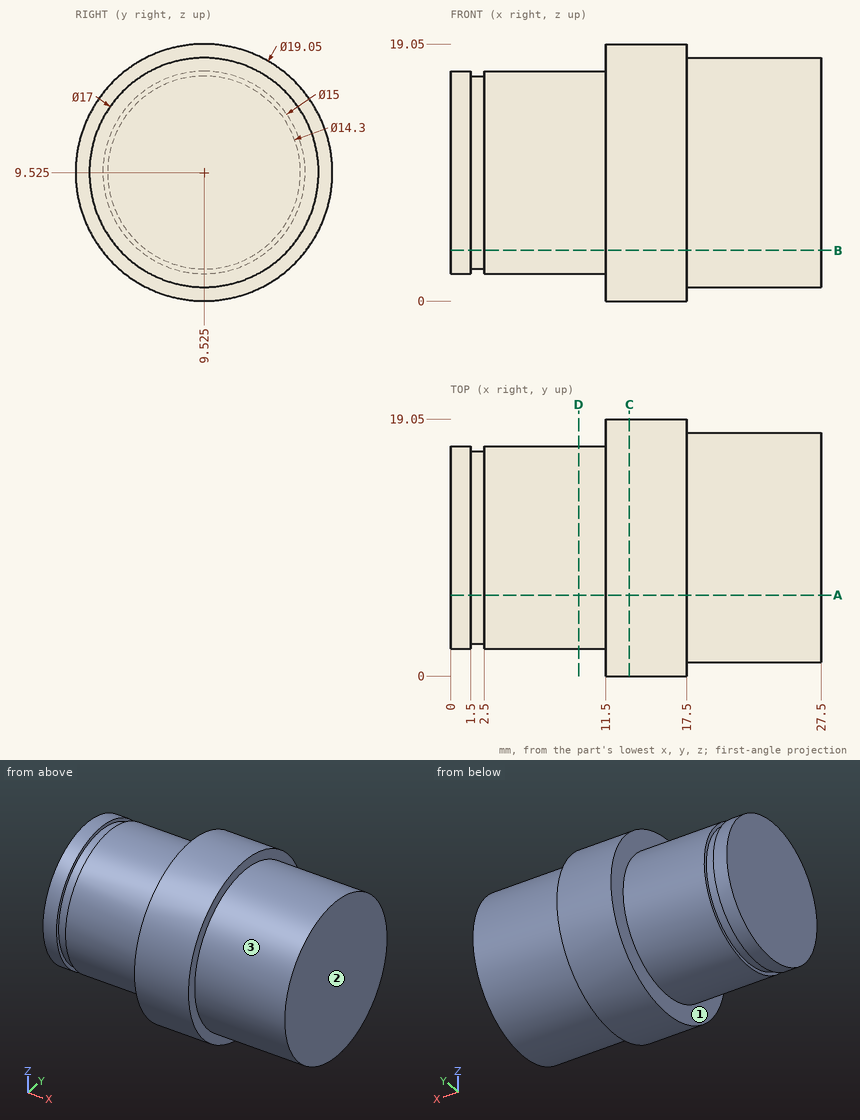
Geometry: see drawing. Coordinates: mm, zero at the bounding-box minimum. A direction names the side the tool comes from. Coordinates: 2 decimals unless noted, no trailing zeros. Loops run counter-clockwise (first coordinate to the right, second up) from the corner with the lowest first, then second, coordinate; pieces in that order, holes last. Notation, with made-up numbers: (-16.5, -16.5) - (17.5, -16.5) arc R22 ccw to (17.5, 19.5) - close; hole circle Ø3 at (3.25, 21). An arc over 180 degrees is marked (long way). Put each result on its own line as item: value. Start each with the question number.
Q1. Cut plane A-A, the plane y = 6. Return loops of the section in (x, z) (3 decimals).
Q2. Set-up query: the marked faces 1, 2 and 3. Return all of +Z, -Z, +X, -X, +Y, -Y with unobstructed straight access to the full face (end or side cutting, diameter ignored); none if empty.
Q3. Pin query (flat end, axial travel): pin 1 Ø5 at (x, z) = (3, 11) entering from -Y (3 decimals); pin 2 Ø8 at (x, y) = (12, 5) entering from -Z; pin 3 Ø8 at (x, y) = (23.5, 4.5) entering from +Z. Return the tip coordinate at first contact, or that it passes through.
Q4. Line query: line 1 (X direction, y = 4.25, z = 16); line 2 (Z direction, x = 10.75, y = 9.25); line 3 (X direction, y = 14.5, z = 2.25). Output: solid intervals per line, ascending.
Q5. Cut plane D-D, the plane x = 9.5. Return loops of the section in (y, z) (3 decimals).
Q6. Cut plane B-B, the plane z = 3.75. Return loops of the section in (x, y).
Q7. Cut plane C-C, the plane x = 13.25. Return loops of the section in (y, z) (3 decimals), and give its area (3 significant figures).
Filled sheet:
1. outline: (0, 2.905) - (1.5, 2.905) - (1.5, 3.304) - (2.5, 3.304) - (2.5, 2.905) - (11.5, 2.905) - (11.5, 0.676) - (17.5, 0.676) - (17.5, 1.79) - (27.5, 1.79) - (27.5, 17.26) - (17.5, 17.26) - (17.5, 18.374) - (11.5, 18.374) - (11.5, 16.145) - (2.5, 16.145) - (2.5, 15.746) - (1.5, 15.746) - (1.5, 16.145) - (0, 16.145) - close
2. face 1: -X
2. face 2: +Z, -Z, +X, +Y, -Y
2. face 3: +X
3. pin 1: y = 2.025
3. pin 2: z = 0.01
3. pin 3: z = 17.96
4. line 1: 11.5 to 27.5
4. line 2: 2.03 to 17.02
4. line 3: 11.5 to 17.5
5. outline: circle Ø15 at (9.525, 9.525)
6. outline: (0, 4.74) - (1.5, 4.74) - (1.5, 5.31) - (2.5, 5.31) - (2.5, 4.74) - (11.5, 4.74) - (11.5, 1.95) - (17.5, 1.95) - (17.5, 3.29) - (27.5, 3.29) - (27.5, 15.76) - (17.5, 15.76) - (17.5, 17.1) - (11.5, 17.1) - (11.5, 14.31) - (2.5, 14.31) - (2.5, 13.74) - (1.5, 13.74) - (1.5, 14.31) - (0, 14.31) - close
7. outline: circle Ø19.05 at (9.525, 9.525)
7. area: 285 mm²
